```python
from build123d import *

# Parameters (mm, degrees)
SKETCH1_R           = 20
BOSS_EXTRUDE1_DEPTH = 50
SKETCH2_W           = 20
SKETCH2_H           = 5.867462555
SKETCH2_H_2         = 6.829602609
CUT_EXTRUDE1_DEPTH  = 119.98554368


with BuildPart() as part:
    # Sketch1 → Boss-Extrude1 (new body)
    with BuildSketch(Plane(origin=(0, 0, 0), x_dir=(0, 0, -1), z_dir=(1, 0, 0))):
        Polygon((29.524911161, 40.713137988), (-70.475088839, 40.713137988), (-70.475088839, 32.713137988), (-50.079010784, 10.713137988), (-50.079010784, -9.286862012), (-70.475088839, -31.286862012), (-70.475088839, -39.286862012), (29.524911161, -39.286862012), (29.524911161, -31.286862012), (9.128833107, -9.286862012), (9.128833107, 10.713137988), (29.524911161, 32.713137988), align=None)
        with Locations((-20.475088839, 0.713137988)):
            Circle(SKETCH1_R, mode=Mode.SUBTRACT)
    extrude(amount=BOSS_EXTRUDE1_DEPTH)

    # Sketch2 → Cut-Extrude1 (cut, through all)
    with BuildSketch(Plane.XY.offset(70.475088839)):
        with Locations((25, 40.713137989)):
            Rectangle(SKETCH2_W, SKETCH2_H)
        with Locations((25, -31.286862012)):
            Rectangle(SKETCH2_W, SKETCH2_H_2)
    extrude(amount=-CUT_EXTRUDE1_DEPTH, mode=Mode.SUBTRACT)


solid = part.part
```
Geometry check sheet. Reference: the model listing, model coordinates, mm. A direction names the side the tool comes from. Coordinates: 2 decimals unless noted, no trailing zeros. Order: outer loops, then holes, each group sorted by start corner. A loop starts at its lowest first (then second) coordinate and runs counter-clockwise, first axis right, second up. Notation, with made-up numbers: (55, -22) - (60, -22) arc R31 cw to (60, 7) - close; hole circle Ø10 at (12, 45). An arc over 180 degrees is marked (long way). Answer in a Markdown table with one row per item. Add a question column.
1. Gauge pin test, flat ends, axial feed: pin 1 Ø1.5 at (x, y) = (19.5, 26.5) entering from +Z; pin 2 Ø16 at (x, z) = (20, 16.5) entering from +Y; pin 3 Ø12 at (y, z) = (8, 58) entering from +X; pin 4 Ø10 at (x, z) = (26, 2) entering from +Y. Record the tip position at first contact, or that the pin passes through.
2. Section check A-A (z = 43). Enter the section's corners in (x, y).
3. Access from +Z, -Z, +X, -X, +Y, -Y to the whole of each face (thin tool, end or side, straight path). Record for faces 4 (the face through (24.65, -20.13, 60.13)), 5 (the face through (35, -31, 21)), 6 (the face through (35, 39, 21)), 7 (the face through (24.65, -20.44, -19.47)).
4. Section check D-D (y = 16). Enter the section's corners in (x, z), plus the area to 3 significant figures.
5. Material ranges on L1, parallel to Y at x = 31, z = -11.5; L2, parallel to Y at x = 22.5, z = 10.5; L3, parallel to X at y = -33.5, z = -1, recorded low to high. Write a range as [from, to].
6. Section check C-C (z = 16.5). Enter the section's corners in (x, y), plus the area to 3 significant figures.
7. Section check B-B (x = 28.5). Enter the section's corners in (y, z).
8. Draft check along X on faces 1 (the face through (50, 19, 10)), 2 (the face through (25, -35, -29.525)), 3 (the face through (25, -34.702, 21)). Enter one of: +X half, -X half, draft (parallel to the pull), parting line (faces both ways), or undercut.
Data:
| question | item | result |
|---|---|---|
| 1 | pin 1 | stops at z = 65.41 |
| 1 | pin 2 | stops at y = 40.71 |
| 1 | pin 3 | passes through |
| 1 | pin 4 | stops at y = 37.78 |
| 2 | outline | (0, -39.29) - (50, -39.29) - (50, 40.71) - (35, 40.71) - (35, 37.78) - (15, 37.78) - (15, 40.71) - (0, 40.71) - close; hole (15, -34.7) - (35, -34.7) - (35, -27.87) - (15, -27.87) - close |
| 3 | face 4 | +Z, +X, -X |
| 3 | face 5 | +Z, -Z |
| 3 | face 6 | +Z, -Z, +Y |
| 3 | face 7 | -Z, +X, -X |
| 4 | outline | (0, -14.03) - (50, -14.03) - (50, 7.58) - (0, 7.58) - close; (0, 33.37) - (50, 33.37) - (50, 54.98) - (0, 54.98) - close |
| 4 | area | 2,160 mm² |
| 5 | L1 | y = [-39.29, -34.7], [-27.87, -11.84], [13.27, 37.78] |
| 5 | L2 | y = [-39.29, -34.7], [-27.87, -16.62], [18.05, 37.78] |
| 5 | L3 | x = [0, 15], [35, 50] |
| 6 | outline | (0, -39.29) - (50, -39.29) - (50, -18.89) - (0, -18.89) - close; (0, 20.31) - (50, 20.31) - (50, 40.71) - (35, 40.71) - (35, 37.78) - (15, 37.78) - (15, 40.71) - (0, 40.71) - close; hole (15, -34.7) - (35, -34.7) - (35, -27.87) - (15, -27.87) - close |
| 6 | area | 1,840 mm² |
| 7 | outline | (-39.29, -29.52) - (-34.7, -29.52) - (-34.7, 70.48) - (-39.29, 70.48) - close; (-27.87, -26.36) - (-9.29, -9.13) - (10.71, -9.13) - (32.71, -29.52) - (37.78, -29.52) - (37.78, 70.48) - (32.71, 70.48) - (10.71, 50.08) - (-9.29, 50.08) - (-27.87, 67.31) - close; hole circle Ø40 at (0.71, 20.48) |
| 8 | face 1 | +X half |
| 8 | face 2 | draft |
| 8 | face 3 | undercut |
